Read the model definition and answer for the solid it produces. Units are mm, in the model's axes. A direction names the side the tool comes from. Coordinates: 2 decimals unless noted, no trailing zeros. Order: outer loops, then holes, each group sorted by start corner. A loop starts at its lowest first (then second) coordinate and runs counter-clockwise, first axis right, second up. Notation, with made-up numbers: M -38.75,30 L 7.25,30 A22 cw 7.25,38 Z; hole C 30.25,79 d10. An arc over 180 degrees is marked long. Write each question's results on one line, items separated by ' | '.
```python
from build123d import *

# Parameters (mm, degrees)
BOSS_EXTRUDE1_DEPTH   = 2.794
F_6_CLEARANCE_HOLE1_D = 3.7973
CUT_EXTRUDE1_REACH    = 75.469
SKETCH5_R             = 5.08


with BuildPart() as part:
    # Sketch1 → Boss-Extrude1 (new, symmetric)
    with BuildSketch(Plane.XY):
        Polygon((-6.35, 49.53), (-6.35, 43.942), (6.35, 43.942), (6.35, 49.53), (53.975, 49.53), (53.975, -49.53), (-53.975, -49.53), (-53.975, 49.53), align=None)
    extrude(amount=BOSS_EXTRUDE1_DEPTH, both=True)

    # #6 Clearance Hole1 (through all)
    with Locations(Plane(origin=(0, 0, -2.794), x_dir=(-1, 0, 0), z_dir=(0, 0, -1))):
        with Locations((-45.014797213, 37.394797213), (-45.014797213, 23.565202787), (45.014797213, 37.394797213), (45.014797213, 23.565202787)):
            Hole(F_6_CLEARANCE_HOLE1_D / 2)

    # Sketch5 → Cut-Extrude1 (cut, up to next)
    with BuildSketch(Plane(origin=(0, 0, -2.794), x_dir=(-1, 0, 0), z_dir=(0, 0, -1)), mode=Mode.PRIVATE) as cut_extrude1_sk1:
        with Locations((0, 30.48)):
            Circle(SKETCH5_R)
    cut_extrude1_tool1 = extrude(cut_extrude1_sk1.sketch, amount=-CUT_EXTRUDE1_REACH, mode=Mode.PRIVATE) & part.part
    add(cut_extrude1_tool1.solids().sort_by_distance((0, 30.48, -2.794))[0], mode=Mode.SUBTRACT)


solid = part.part
```
(1) For faces 4 (the flat face through (0, 43.942, 0)), 5 (the flat face through (30, 49.53, 0)), determine the directions among +Z, -Z, +X, -X, +Y, -Y from which every point of the face is accessible in a straight line to the end or side of a thin tool.
Conclusion:
face 4: +Z, -Z, +Y | face 5: +Z, -Z, +X, -X, +Y
(2) Given pin 1 (1.7 mm diameter, centred on x = 2.5, z = 1, fed in from +Y); pin 2 (4.5 mm diameter, centred on x = 45.01, y = 37.39, fed in from +Z), each flat-ended and moving along its own axis, determine where each tip first touches the part or whether it passes through.
Conclusion:
pin 1: y = 43.94 | pin 2: z = 2.79
(3) The part is cut by section C-C, the plane z = 0.65. Write down the section's boundary in (x, y) (3 decimals).
Conclusion:
outline: M -53.975,-49.53 L 53.975,-49.53 L 53.975,49.53 L 6.35,49.53 L 6.35,43.942 L -6.35,43.942 L -6.35,49.53 L -53.975,49.53 Z; hole C -45.015,23.565 d3.797; hole C -45.015,37.395 d3.797; hole C 0,30.48 d10.16; hole C 45.015,23.565 d3.797; hole C 45.015,37.395 d3.797
(4) The part is cut by section B-B, the plane y = 30.48. Write down the section's boundary in (x, z) (3 decimals).
Conclusion:
outline: M -53.975,-2.794 L -5.08,-2.794 L -5.08,2.794 L -53.975,2.794 Z; M 5.08,-2.794 L 53.975,-2.794 L 53.975,2.794 L 5.08,2.794 Z
(5) The mould has two halves that part along X. Classify faces 1 (the flat face through (-53.975, -1, 0)), 2 (the flat face through (1, -49.53, 0)), 3 (the cylindrical face through (1.1, 25.52, -0.04)): pulls with the +X half, pulls with the -X half, needs draft (parallel to the pull), parting line crosses it, or undercut.
Conclusion:
face 1: pulls with the -X half | face 2: needs draft | face 3: undercut
(6) The part is cut by section A-A, the plane x = 0. Write down the section's boundary in (y, z), then the cut area to 3 significant figures.
Conclusion:
outline: M -49.53,-2.79 L 25.4,-2.79 L 25.4,2.79 L -49.53,2.79 Z; M 35.56,-2.79 L 43.94,-2.79 L 43.94,2.79 L 35.56,2.79 Z | area: 466 mm²
(7) Straight lines are drawn through the part: line 1 (Y direction, x = 0, z = 0.6); line 2 (X direction, y = 22, z = 2.4) (3 decimals); line 3 (Y direction, x = -3, z = -1.75). For each, find the intervals that lie inside material, in ascending order.
Conclusion:
line 1: -49.53 to 25.4, 35.56 to 43.94 | line 2: -53.975 to -46.09, -43.94 to 43.94, 46.09 to 53.975 | line 3: -49.53 to 26.38, 34.58 to 43.94
